The model under review builds one solid part; all positions refer to its coordinate system, in mm. Coordinates: 2 decimals unless noted, no trailing zeros. Write each loop counter-clockwise with the first axis right and the second up, starting at its lowest first coordinate (ties: lowest second). Pieces come first, ordered by that corner, then holes. Notation, with made-up numbers: (-28, 57.25) - (-5, 57.25) arc R18 cw to (-5, 74.25) - close; hole circle Ø1 at (12, 79.5). An arc over 180 degrees is marked (long way). Return JSON: item names as keys, results as strings. Group by question number.
(1) To check wall thickness, follow L1, parallel to Y at x = -48, z = 2.3; L2, parallel to X at y = 23, z = 1.7; L3, parallel to Y at x = 0.5, z = 1.5. State the ranges of each line that lie inside material, in increasing order. Write a range as from..to.
(2) We need section D-D on y = 0. State the section outline as (x, z) points, then the cut area to 3 significant figures.
(3) We need section C-C on x = -48. State the section outline as (y, z) points, then the cut area to 4 significant figures.
(4) We need section A-A on x = 48.5. State the section outline as (y, z) points.
(5) We need section B-B on y = -12. State the section outline as (x, z) points.
(6) For pin 1 Ø0.9 at (y, z) = (-2, 1.5) entering from -X; pin 2 Ø0.9 at (x, z) = (63, 1.5) entering from -Y; pin 3 Ø8 at (x, y) = (0, 0) entering from -Z, all flat-tipped, find the tip position at first contact; note any pin that passes through.
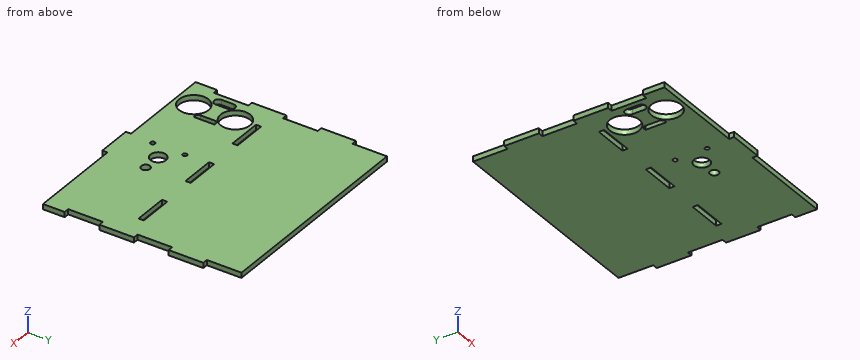
```python
from build123d import *

# Parameters (mm, degrees)
SKETCH1_R           = 8.5
SKETCH1_R_2         = 4.5
SKETCH1_R_3         = 2.5
SKETCH1_R_4         = 1.25
SKETCH1_W           = 20
SKETCH1_H           = 3
BOSS_EXTRUDE1_DEPTH = 3


with BuildPart() as part:
    # Sketch1 → Boss-Extrude1 (new body)
    with BuildSketch(Plane.XY):
        Polygon((-10, -22.5), (-65, -22.5), (-65, -10), (-62, -10), (-62, 10), (-65, 10), (-65, 22.5), (-65, 30), (-62, 30), (-62, 50), (-65, 50), (-65, 70), (-62, 70), (-62, 90), (62, 90), (62, 70), (65, 70), (65, 50), (62, 50), (62, 30), (65, 30), (65, 22.5), (65, 10), (62, 10), (62, -10), (65, -10), (65, -22.5), (10, -22.5), (10, -25.5), (-10, -25.5), align=None)
        with Locations((-48, 12)):
            Circle(SKETCH1_R, mode=Mode.SUBTRACT)
        with Locations((-48, -12)):
            Circle(SKETCH1_R, mode=Mode.SUBTRACT)
        Circle(SKETCH1_R_2, mode=Mode.SUBTRACT)
        with Locations((10.75, 0)):
            Circle(SKETCH1_R_3, mode=Mode.SUBTRACT)
        with Locations((-9, 9.25)):
            Circle(SKETCH1_R_4, mode=Mode.SUBTRACT)
        with Locations(Location((-9, -9.25, 0), (0, 0, 180))):
            Circle(SKETCH1_R_4, mode=Mode.SUBTRACT)
        with BuildLine():
            Line((-54, 3.5), (-54, -3.5))
            ThreePointArc((-54, -3.5), (-56.5, -6), (-59, -3.5))
            Line((-59, -3.5), (-59, 3.5))
            ThreePointArc((-59, 3.5), (-56.5, 6), (-54, 3.5))
        make_face(mode=Mode.SUBTRACT)
        with BuildLine():
            Line((-39, -6), (-40, -6))
            ThreePointArc((-40, -6), (-41.414213562, -5.414213562), (-42, -4))
            Line((-42, -4), (-42, 4))
            ThreePointArc((-42, 4), (-41.414213562, 5.414213562), (-40, 6))
            Line((-40, 6), (-39, 6))
            Line((-39, 6), (-39, -6))
        make_face(mode=Mode.SUBTRACT)
        with Locations((40, 24)):
            Rectangle(SKETCH1_W, SKETCH1_H, mode=Mode.SUBTRACT)
        with Locations((0, 24)):
            Rectangle(SKETCH1_W, SKETCH1_H, mode=Mode.SUBTRACT)
        with Locations((-40, 24)):
            Rectangle(SKETCH1_W, SKETCH1_H, mode=Mode.SUBTRACT)
    extrude(amount=BOSS_EXTRUDE1_DEPTH)


solid = part.part
```
Ans:
{
 "1": {"L1": "-22.5..-20.5, -3.5..3.5, 20.5..22.5, 25.5..90", "L2": "-65..-50, -30..-10, 10..30, 50..65", "L3": "-25.5..-4.47, 4.47..22.5, 25.5..90"},
 "2": {"outline": "(-62, 0) - (-59, 0) - (-59, 3) - (-62, 3) - close; (-54, 0) - (-42, 0) - (-42, 3) - (-54, 3) - close; (-39, 0) - (-4.5, 0) - (-4.5, 3) - (-39, 3) - close; (4.5, 0) - (8.25, 0) - (8.25, 3) - (4.5, 3) - close; (13.25, 0) - (62, 0) - (62, 3) - (13.25, 3) - close", "area": "306 mm²"},
 "3": {"outline": "(-22.5, 0) - (-20.5, 0) - (-20.5, 3) - (-22.5, 3) - close; (-3.5, 0) - (3.5, 0) - (3.5, 3) - (-3.5, 3) - close; (20.5, 0) - (22.5, 0) - (22.5, 3) - (20.5, 3) - close; (25.5, 0) - (90, 0) - (90, 3) - (25.5, 3) - close", "area": "226.5 mm²"},
 "4": {"outline": "(-22.5, 0) - (22.5, 0) - (22.5, 3) - (-22.5, 3) - close; (25.5, 0) - (90, 0) - (90, 3) - (25.5, 3) - close"},
 "5": {"outline": "(-65, 0) - (-56.5, 0) - (-56.5, 3) - (-65, 3) - close; (-39.5, 0) - (65, 0) - (65, 3) - (-39.5, 3) - close"},
 "6": {"pin 1": "x = -62", "pin 2": "y = -22.5", "pin 3": "through"}
}
